Design review of the part built by this model. Coordinates are the model's own, in mm. Round coordinates to 2 decimals unless told otherwise and drop trailing zeros. Order: outer loops, then holes, each group sorted by start corner. A loop starts at its lowest first (then second) coordinate and runs counter-clockwise, first axis right, second up.
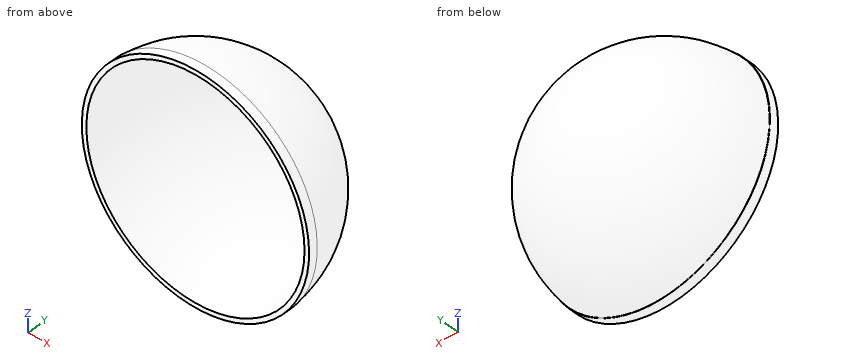
from build123d import *

# Parameters (mm, degrees)
REVOLVE1_ANGLE      = 180
SHELL1_T            = -1.27
SKETCH6_R           = 31.75
SKETCH6_R_2         = 30.48
BOSS_EXTRUDE1_DEPTH = 2.54


with BuildPart() as part:
    # Sketch1 → Revolve1 (revolve)
    with BuildSketch(Plane(origin=(0, 0, 0), x_dir=(1, 0, 0), z_dir=(0, 1, 0))):
        with BuildLine():
            Line((0, 31.75), (0, -31.75))
            ThreePointArc((0, -31.75), (31.75, 0), (0, 31.75))
        make_face()
    revolve(axis=Axis((0, 0, -31.75), (0, 0, 1)), revolution_arc=REVOLVE1_ANGLE)

    # Shell1
    shell1_openings = [part.faces().sort_by_distance(p)[0] for p in [
        (0, 0, 0),
    ]]
    offset(amount=SHELL1_T, openings=shell1_openings)

    # Sketch6 → Boss-Extrude1 (add)
    with BuildSketch(Plane(origin=(0, 0, 0), x_dir=(1, 0, 0), z_dir=(0, 1, 0))):
        with Locations(Location((0, 0, 0), (0, 0, 270))):
            Circle(SKETCH6_R)
        Circle(SKETCH6_R_2, mode=Mode.SUBTRACT)
    extrude(amount=BOSS_EXTRUDE1_DEPTH)


solid = part.part
1) To check wall thickness, follow line 1 along X through (y, z) = (5, 23.5); line 2 along Z through (x, y) = (5, 27); line 3 along X through (y, z) = (2.5, -24). State the ranges of each line that lie inside material, in increasing order.
Results:
line 1: x = -20.76 to -18.76, 18.76 to 20.76
line 2: z = -15.94 to -13.23, 13.23 to 15.94
line 3: x = -20.79 to -18.62, 18.62 to 20.79
2) Take a section at A-A on z = 0. Give the boundary of the cut face in (x, y), plus the area to 3 significant figures.
Results:
outline: (-31.75, 0) - (-30.48, 0) arc R30.48 cw to (30.48, 0) - (31.75, 0) - (31.75, 2.54) - (31.65, 2.54) arc R31.75 ccw to (-31.65, 2.54) - (-31.75, 2.54) - close
area: 124 mm2
3) Clearance check with flat-ended pins moving along their axes: P1, Ø4, axis at y = 12, z = -1.5, coming from the -X side; P2, Ø10, axis at x = 4.5, y = 18, coming from the +Z side; P3, Ø4, axis at x = -11.5, z = 21.5, coming from the +Y side. State where each tip first meets the part, or that it passes through.
Results:
P1: stops at x = -30.1
P2: stops at z = 28.71
P3: stops at y = 22.52
4) Take a section at C-C on y = 15. Give the boundary of the cut face in (x, z).
Results:
outline: circle Ø55.97 at (0, 0); hole circle Ø53.07 at (0, 0)
5) Take a section at B-B on x = 0. Give the boundary of the cut face in (y, z), plus the area to 3 significant figures.
Results:
outline: (0, -31.75) - (2.54, -31.75) - (2.54, -31.65) arc R31.75 ccw to (2.54, 31.65) - (2.54, 31.75) - (0, 31.75) - (0, 30.48) arc R30.48 cw to (0, -30.48) - close
area: 124 mm2
